Here's the drawing with two shaded views (mm, measured from the low corner). I have some questions. Coordinates: 2 decimals unless noted, no trailing zeros. Loops run counter-clockwise (first coordinate to the right, second up) from the corner with the lowest first, then second, coordinate; pieces in that order, holes last. Notation, with made-up numbers: (-13, -13) -> (38, -13) arc R13 cw to (38, -6) -> close; hole circle Ø11 at (17.5, 85). An arc over 180 degrees is marked (long way). Answer as a JSON object with one key per item and string values. Group by question number.
1) I want a section at C-C (y = 10). Write out the boundary of the cut face in (x, z).
2) I need wall thicknesses on probe 1 along Y at (x, z) = (5, 1.7); probe 2 along X at (y, z) = (32, 1.05) (1 decimal); probe 3 along Y at (x, z) = (50, 2.1). Which ranges of each line are inside material? Lowest first, please. Write a range as [from, to].
3) I want a section at D-D (z = 1.1). Count the separate pieces of the cut face and the enclosed holes in it, then the cut area to 3 significant figures.
4) I want a section at B-B (y = 5). Write out the boundary of the cut face in (x, z), then the cut area to 3 significant figures.
5) I want a section at A-A (x = 5). Write out the boundary of the cut face in (y, z).
6) I'm going to push flat-ended pins straight in: pin 1 (0.7 mm diameter, centred on y = 33, z = 2, fed in from +X); pin 2 (1 mm diameter, centred on x = 36.5, z = 0.5, fed in from -Y). Where does each tip first touch, or does it pass through?
7) If we mould it in two halves opening along Z, with no side actions, what happens to the marked faces 1 and 2? For each: +Z half, -Z half, draft (parallel to the pull), parting line (faces both ways), or undercut.
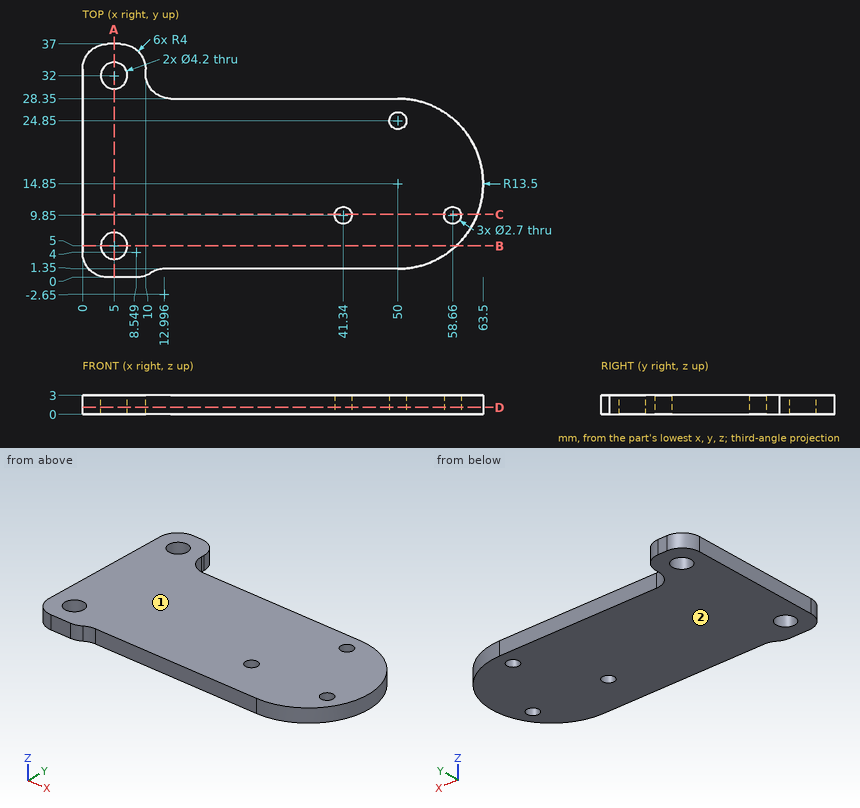
Determined:
{
 "1": {"outline": "(0, 0) -> (40, 0) -> (40, 3) -> (0, 3) -> close; (42.68, 0) -> (57.32, 0) -> (57.32, 3) -> (42.68, 3) -> close; (60, 0) -> (62.6, 0) -> (62.6, 3) -> (60, 3) -> close"},
 "2": {"probe 1": "[0, 2.9], [7.1, 29.9], [34.1, 37]", "probe 2": "[0, 2.9], [7.1, 10]", "probe 3": "[1.35, 23.5], [26.2, 28.35]"},
 "3": {"separate pieces": "1", "enclosed holes": "5", "area": "1,690 mm^2"},
 "4": {"outline": "(0, 0) -> (2.9, 0) -> (2.9, 3) -> (0, 3) -> close; (7.1, 0) -> (59.23, 0) -> (59.23, 3) -> (7.1, 3) -> close", "area": "165 mm^2"},
 "5": {"outline": "(0, 0) -> (2.9, 0) -> (2.9, 3) -> (0, 3) -> close; (7.1, 0) -> (29.9, 0) -> (29.9, 3) -> (7.1, 3) -> close; (34.1, 0) -> (37, 0) -> (37, 3) -> (34.1, 3) -> close"},
 "6": {"pin 1": "x = 10", "pin 2": "y = 1.35"},
 "7": {"face 1": "+Z half", "face 2": "-Z half"}
}
